from build123d import *

# Parameters (mm, degrees)
F0_W     = 17.78
F0_H     = 17.78
F1_DEPTH = 7.62
F3_W     = 5.08
F3_H     = 22.724437993
F5_R     = 4.445
F5_R_2   = 3.1115
F6_DEPTH = 10.16
F7_DEPTH = 25.4
F8_DEPTH = 10.16


# Not quite as in the source:
# - a fillet or chamfer that OpenCascade refuses, or shapes differently, is made with other operations: its cross-section is extruded or revolved along the edge and cut away or added


with BuildPart() as f1:
    # F0 (on Top) → F1 (new body)
    with BuildSketch(Plane.XY):
        with Locations((8.89, 8.89)):
            Rectangle(F0_W, F0_H)
    extrude(amount=F1_DEPTH)

    # F3 (on offset) → F4 (revolve, cut)
    with BuildSketch(Plane(origin=(0, 0, -19.05), x_dir=(1, 0, 0), z_dir=(0, 0, -1))):
        with Locations((-12.065, -8.8908823673)):
            Rectangle(F3_W, F3_H)
    revolve(axis=Axis((8.89, 12.1113763889, -19.05), (0, 1, 0)), mode=Mode.SUBTRACT)

    # F5 (on face) → F6 (join)
    with BuildSketch(Plane.XY.offset(7.62)):
        with Locations((8.89, 8.89)):
            Circle(F5_R)
        with Locations((8.89, 8.89)):
            Circle(F5_R_2, mode=Mode.SUBTRACT)
    extrude(amount=F6_DEPTH)

    # F7 (cut): a face of the model
    f7_faces = [f1.faces().sort_by_distance(p)[0] for p in [
        (8.89, 8.89, 7.62),
    ]]
    extrude(f7_faces, amount=-F7_DEPTH, mode=Mode.SUBTRACT)

    # F5 (on face) → F8 (join)
    with BuildSketch(Plane.XY.offset(7.62)):
        with Locations((8.89, 8.89)):
            Circle(F5_R)
        with Locations((8.89, 8.89)):
            Circle(F5_R_2, mode=Mode.SUBTRACT)
    extrude(amount=-F8_DEPTH)

    # F9: chamfer of 1.778 on 1 edges, made by hand

    # F9_s1 → F9_t2 (revolve, cut)
    with BuildSketch(Plane.XZ.offset(-8.89)):
        Polygon((13.7795, 17.78), (12.0015, 16.002), (12.0015, 17.78), align=None)
    revolve(axis=Axis((8.89, 8.89, 17.78), (0, 0, 1)), mode=Mode.SUBTRACT)


solid = f1.part
Build history of the part. All positions in model axes, mm. A direction names the side the tool comes from. Round coordinates to 2 decimals unless told otherwise and drop trailing zeros. Order: outer loops, then holes, each group sorted by start corner. A loop starts at its lowest first (then second) coordinate and runs counter-clockwise, first axis right, second up. Notation, with made-up numbers: M 39,59.25 L 45,59.25 A22 ccw 45,90.25 Z; hole C 84,34.25 d1. An arc over 180 degrees is marked long. Use CSV: the item, a comma, the result in double quotes. Start each with the question number.
(1) Cut at B-B on z = 9.5. List the corners of the cut face in (x, y) (1 decimal).
(2) Cut at D-D on y = 14.25. List the corners of the cut face in (x, z) (3 decimals).
(3) Cut at A-A on x = 8.89. List the corners of the cut face in (y, z) (1 decimal), then the cut area to 3 significant figures.
(4) Tool access for faces 1 (the face through (6.739, 4.814, 4.346)), 2 (the face through (4.8, 11, 7.62)), 3 (the face through (10, 12, -2.54)): list every direction of +Z, -Z, +X, -X, +Y, -Y with a clear straight run to the whole face (end or side of a thin tool).
(5) Drill centre lines: probe 1 along Y at (x, z) = (8.89, 9.5) (1 decimal); probe 2 along Y at (x, z) = (8.89, 7.5). Where is each one in solid material? Low to high.
(6) Flat gauge pins, fed straight in: P1, Ø1, axis at y = 7, z = 9, coming from the -X side; P2, Ø4, axis at x = 9, z = 2, coming from the -Y side (3 decimals); P3, Ø1, axis at x = 14, y = 9, coming from the +Z side. Where does each tip first touch, or does it go through?
Findings:
1,outline,"C 8.9,8.9 d8.9; hole C 8.9,8.9 d6.2"
2,outline,"M 0,2.698 A23.495 cw 17.78,2.698 L 17.78,7.62 L 0,7.62 Z"
3,outline,"M 0,4.4 L 4.4,4.4 L 4.4,-2.5 L 5.8,-2.5 L 5.8,16 L 4.4,17.3 L 4.4,7.6 L 0,7.6 Z; M 12,-2.5 L 13.3,-2.5 L 13.3,4.4 L 17.8,4.4 L 17.8,7.6 L 13.3,7.6 L 13.3,17.3 L 12,16 Z"
3,area,"79.5 mm^2"
4,face 1,"-Z"
4,face 2,"+Z"
4,face 3,"-Z, +X, -X, +Y, -Y"
5,probe 1,"y = 4.4 to 5.8, 12 to 13.3"
5,probe 2,"y = 0 to 5.78, 12 to 17.78"
6,P1,"stops at x = 4.67"
6,P2,"stops at y = 4.445"
6,P3,"stops at z = 7.62"
